Check sheet for the modelled part. Datum: model origin and axes. Units: mm. Face numbers are marked on the shaded views. A direction names the side the tool comes from. Give positions to 0.01 mm unless a question says otherwise; leave off trailing zeros. Loops run counter-clockwise (first coordinate to the right, second up) from the corner with the lowest first, then second, coordinate; pieces in that order, holes last.
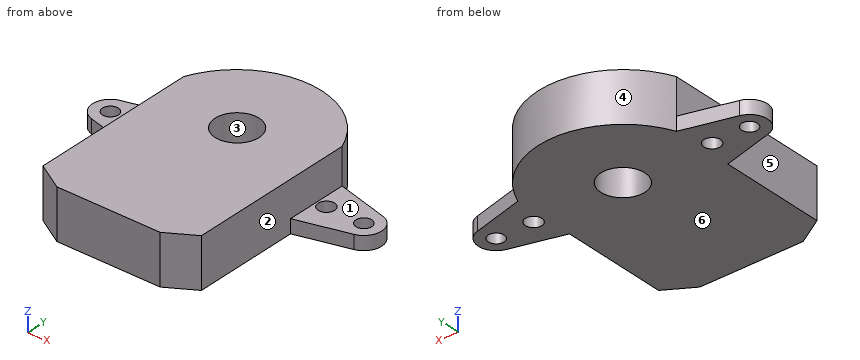
```python
from build123d import *

# Parameters (mm, degrees)
SKETCH_1_R          = 4
SKETCH_1_R_2        = 1.435
SKETCH_1_R_3        = 1.5
EXTRUDE_1_DEPTH     = 9
CUT_EXTRUDE_START   = -6.5
CUT_EXTRUDE_1_DEPTH = 6.5
CHAMFER_1_SIZE      = 5
CHAMFER_1_SIZE2     = 3
CHAMFER_2_SIZE      = 3
CHAMFER_2_SIZE2     = 5


with BuildPart() as part:
    # ｽｹｯﾁ1 → ﾎﾞｽ - 押し出し1 (new body)
    with BuildSketch(Plane.XY):
        with BuildLine():
            Line((14.385, -28.04), (-14.385, -28.04))
            Line((-14.385, -28.04), (-14.385, -5.612501624))
            Line((-14.385, -5.612501624), (-23.834680852, -3.131361508))
            ThreePointArc((-23.834680852, -3.131361508), (-26.25, 0), (-23.834680852, 3.131361508))
            Line((-23.834680852, 3.131361508), (-14.385, 5.612501624))
            ThreePointArc((-14.385, 5.612501624), (0, 15.34), (14.385, 5.612501624))
            Line((14.385, 5.612501624), (23.834680852, 3.131361508))
            ThreePointArc((23.834680852, 3.131361508), (26.25, 0), (23.834680852, -3.131361508))
            Line((23.834680852, -3.131361508), (14.385, -5.612501624))
            Line((14.385, -5.612501624), (14.385, -28.04))
        make_face()
        Circle(SKETCH_1_R, mode=Mode.SUBTRACT)
        with Locations((-23.0125, 0)):
            Circle(SKETCH_1_R_2, mode=Mode.SUBTRACT)
        with Locations((23.0125, 0)):
            Circle(SKETCH_1_R_2, mode=Mode.SUBTRACT)
        with Locations((-16.215, 0)):
            Circle(SKETCH_1_R_3, mode=Mode.SUBTRACT)
        with Locations(Location((16.215, 0, 0), (0, 0, 180))):
            Circle(SKETCH_1_R_3, mode=Mode.SUBTRACT)
    extrude(amount=EXTRUDE_1_DEPTH)

    # ｽｹｯﾁ2 → ｶｯﾄ - 押し出し1 (cut)
    with BuildSketch(Plane.XY.offset(9).offset(CUT_EXTRUDE_START)):
        with BuildLine():
            Line((-14.385, 5.612501624), (-23.834680852, 3.131361508))
            ThreePointArc((-23.834680852, 3.131361508), (-26.25, 0), (-23.834680852, -3.131361508))
            Line((-23.834680852, -3.131361508), (-14.385, -5.612501624))
            Line((-14.385, -5.612501624), (-14.385, 5.612501624))
        make_face()
        with BuildLine():
            Line((14.385, -5.612501624), (14.385, 5.612501624))
            Line((14.385, 5.612501624), (23.834680852, 3.131361508))
            ThreePointArc((23.834680852, 3.131361508), (26.25, 0), (23.834680852, -3.131361508))
            Line((23.834680852, -3.131361508), (14.385, -5.612501624))
        make_face()
    extrude(amount=CUT_EXTRUDE_1_DEPTH, mode=Mode.SUBTRACT)

    # 面取り1
    chamfer_1_edges = [part.edges().sort_by_distance(p)[0] for p in [
        (14.385, -28.04, 4.5),
    ]]
    chamfer_1_side = [part.faces().sort_by_distance(p)[0] for p in [
        (0, -28.04, 4.5),
    ]]
    chamfer(chamfer_1_edges, length=CHAMFER_1_SIZE, length2=CHAMFER_1_SIZE2, reference=chamfer_1_side[0])

    # 面取り2
    chamfer_2_edges = [part.edges().sort_by_distance(p)[0] for p in [
        (-14.385, -28.04, 4.5),
    ]]
    chamfer_2_side = [part.faces().sort_by_distance(p)[0] for p in [
        (-14.385, -12.358852788, 4.831877112),
    ]]
    chamfer(chamfer_2_edges, length=CHAMFER_2_SIZE, length2=CHAMFER_2_SIZE2, reference=chamfer_2_side[0])


solid = part.part
```
(1) Section check B-B on y = 0. Give the number of separate pieces and of enclosed holes in the cut face, plus the area to 3 significant figures.
(2) Gauge pin test, flat ends, axial feed: pin 1 Ø2.5 at (x, y) = (16.215, 0) entering from +Z; pin 2 Ø1 at (y, z) = (8.5, 3) entering from -X; pin 3 Ø2.5 at (y, z) = (-9.5, 4) entering from -X (3 decimals); pin 4 Ø1 at (y, z) = (7, 3.5) entering from +X. Record the tip position at first contact, or that the pin passes through.
(3) Access from +Z, -Z, +X, -X, +Y, -Y to the whole of each face (thin tool, end or side, straight path). Record for the marked faces 5 and 6.
(4) Release check for a two-part mould opening along X. For the marked faces 1, 2, 3 and 4 record: pulls with the +X half, pulls with the -X half, needs draft (parallel to the pull), parting line crosses it, or undercut.
(5) Section check D-D on y = -12.5. Record the boundary of the cut face in (x, z) (3 decimals), plus the area to 3 significant figures.
(6) Material ranges on line 1 (Y direction, x = 0, z = 3.5); line 2 (X direction, y = -6, z = 8.5) (3 decimals); line 3 (Y direction, x = 24, z = 1), recorded low to high.
(7) Section check A-A on x = 0. Record the boundary of the cut face in (y, z).
(8) Section check C-C on z = 8. Record the boundary of the cut face in (x, y) (1 decimal), plus the area to 3 significant figures.
Computed values:
1. separate pieces: 6
1. enclosed holes: 0
1. area: 217 mm2
2. pin 1: passes through
2. pin 2: stops at x = -13.18
2. pin 3: stops at x = -14.385
2. pin 4: stops at x = 14
3. face 5: +Z, -X, -Y
3. face 6: -Z, +X, -X, +Y, -Y
4. face 1: needs draft
4. face 2: pulls with the +X half
4. face 3: undercut
4. face 4: parting line crosses it
5. outline: (-14.385, 0) - (14.385, 0) - (14.385, 9) - (-14.385, 9) - close
5. area: 259 mm2
6. line 1: y = -28.04 to -4, 4 to 15.34
6. line 2: x = -14.385 to 14.385
6. line 3: y = -3.08 to -1.04, 1.04 to 3.08
7. outline: (-28.04, 0) - (-4, 0) - (-4, 9) - (-28.04, 9) - close; (4, 0) - (15.34, 0) - (15.34, 9) - (4, 9) - close
8. outline: (-14.4, -25) - (-9.4, -28) - (9.4, -28) - (14.4, -25) - (14.4, 5.6) arc R15.5 ccw to (-14.4, 5.6) - close; hole circle Ø8 at (0, 0)
8. area: 1,110 mm2
